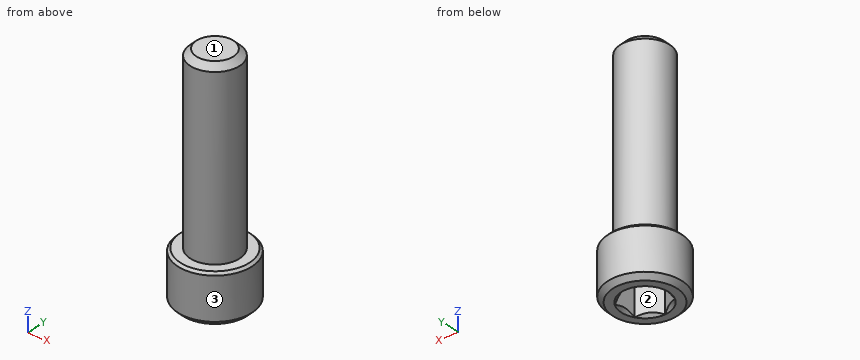
from build123d import *

# Parameters (mm, degrees)
SKETCH1_R          = 4.7625
EXTRUDE1_DEPTH     = 34.925
SKETCH6_R          = 7.14375
EXTRUDE2_DEPTH     = 9.525
CUT_EXTRUDE1_DEPTH = 5.953125
SKETCH8_R          = 4.582717762
CUT_EXTRUDE2_DEPTH = 0.9525
CUT_EXTRUDE2_DRAFT = -45
CHAMFER1_SIZE      = 0.9525
CHAMFER2_SIZE      = 0.47625
CHAMFER3_SIZE      = 1.190625


with BuildPart() as part:
    # Sketch1 → Extrude1 (new body)
    with BuildSketch(Plane.XY):
        Circle(SKETCH1_R)
    extrude(amount=-EXTRUDE1_DEPTH)

    # Sketch6 → Extrude2 (add)
    with BuildSketch(Plane(origin=(0, 0, -34.925), x_dir=(-1, 0, 0), z_dir=(0, 0, -1))):
        with Locations(Location((0, 0, 0), (0, 0, 180))):
            Circle(SKETCH6_R)
    extrude(amount=EXTRUDE2_DEPTH)

    # Sketch7 → Cut-Extrude1 (cut)
    with BuildSketch(Plane(origin=(0, 0, -44.45), x_dir=(-1, 0, 0), z_dir=(0, 0, -1))):
        Polygon((0, 4.582717762), (-3.96875, 2.291358881), (-3.96875, -2.291358881), (0, -4.582717762), (3.96875, -2.291358881), (3.96875, 2.291358881), align=None)
    extrude(amount=-CUT_EXTRUDE1_DEPTH, mode=Mode.SUBTRACT)


with BuildPart() as cut_extrude2_tool:
    # Sketch8 → Cut-Extrude2 (with draft: the straight prism first)
    with BuildSketch(Plane(origin=(0, 0, -44.45), x_dir=(-1, 0, 0), z_dir=(0, 0, -1))):
        Circle(SKETCH8_R)
    extrude(amount=-CUT_EXTRUDE2_DEPTH)
    # Cut-Extrude2: the draft: its side faces are tilted about the plane it starts from
    cut_extrude2_sides = [cut_extrude2_tool.faces().sort_by_distance(p)[0] for p in [
        (4.582717762, 0, -43.97375),
    ]]
    draft(cut_extrude2_sides, Plane(origin=(0, 0, -44.45), x_dir=(-1, 0, 0), z_dir=(0, 0, -1)), CUT_EXTRUDE2_DRAFT)


with BuildPart() as part_1:
    add(part.part)

    # Cut-Extrude2: cut by cut_extrude2_tool
    add(cut_extrude2_tool.part, mode=Mode.SUBTRACT)

    # Chamfer1
    chamfer1_edges = [part_1.edges().sort_by_distance(p)[0] for p in [
        (-7.14375, 0, -44.45),
    ]]
    chamfer(chamfer1_edges, length=CHAMFER1_SIZE)

    # Chamfer2
    chamfer2_edges = [part_1.edges().sort_by_distance(p)[0] for p in [
        (-7.14375, 0, -34.925),
    ]]
    chamfer(chamfer2_edges, length=CHAMFER2_SIZE)

    # Chamfer3
    chamfer3_edges = [part_1.edges().sort_by_distance(p)[0] for p in [
        (-4.7625, 0, 0),
    ]]
    chamfer(chamfer3_edges, length=CHAMFER3_SIZE)


solid = part_1.part
Could you check a few things on this model? Use its own coordinates, in mm. Face numbers are marked on the shaded views. Give positions to 0.01 mm unless a question says otherwise; leave off trailing zeros. Order: outer loops, then holes, each group sorted by start corner. A loop starts at its lowest first (then second) coordinate and runs counter-clockwise, first axis right, second up. Notation, with made-up numbers: (-20.75, -33) -> (-12.75, -33) arc R22 cw to (-12.75, 6) -> close; hole circle Ø5 at (-22.5, 22.5). An arc over 180 degrees is marked (long way). Answer in a Markdown table with one row per item. Add a question column.
Item 1: Imagine slicing it at B-B (z = -36). List the corners of the cut face in (x, y) for me.
Item 2: I'm going to push flat-ended pins straight in: P1, Ø1.5, axis at x = -4, y = -1, coming from the -Z side; P2, Ø1, axis at x = 2, z = -36.5, coming from the -Y side; P3, Ø2, axis at x = 2.5, y = -5.5, coming from the +Z side (3 decimals); P4, Ø2, axis at x = -0.5, z = -25.5, coming from the -Y side. Where does each tip first touch, or does it pass through?
Item 3: Imagine slicing it at C-C (z = -17.5). List the corners of the cut face in (x, y) for me (1 decimal), and give its area (3 significant figures).
Item 4: We'd pull the mould along X, two halves only. Please class the marked faces 1, 2 and 3: pulls with the +X half, pulls with the -X half, needs draft (parallel to the pull), parting line crosses it, or undercut.
Item 5: Please list where these lines run through material, in increasing order: probe 1 along Z at (x, y) = (-1.75, -0.5); probe 2 along Y at (x, z) = (0, -16); probe 3 along Z at (x, y) = (-4.75, -3.75) (3 decimals).
Result:
| question | item | result |
|---|---|---|
| 1 | outline | circle Ø14.29 at (0, 0) |
| 2 | P1 | z = -44.45 |
| 2 | P2 | y = -6.98 |
| 2 | P3 | z = -34.925 |
| 2 | P4 | y = -4.76 |
| 3 | outline | circle Ø9.5 at (0, 0) |
| 3 | area | 71.3 mm2 |
| 4 | face 1 | needs draft |
| 4 | face 2 | undercut |
| 4 | face 3 | parting line crosses it |
| 5 | probe 1 | -38.5 to 0 |
| 5 | probe 2 | -4.76 to 4.76 |
| 5 | probe 3 | -44.45 to -34.925 |
